```python
from build123d import *

# Parameters (mm, degrees)
BOSS_EXTRUDE1_DEPTH = 30
SKETCH2_R           = 1.5
CUT_EXTRUDE1_DEPTH  = 3
SKETCH3_R           = 1.5
SKETCH3_W           = 15
SKETCH3_H           = 45
CUT_EXTRUDE2_DEPTH  = 3
SKETCH4_W           = 30
SKETCH4_H           = 3
BOSS_EXTRUDE2_DEPTH = 4.75
SKETCH5_R           = 1.5
CUT_EXTRUDE3_DEPTH  = 3
BOSS_EXTRUDE3_DEPTH = 3
BOSS_EXTRUDE4_DEPTH = 3
FILLET1_R           = 1


with BuildPart() as part:
    # Sketch1 → Boss-Extrude1 (new body)
    with BuildSketch(Plane(origin=(0, 0, 0), x_dir=(0, 0, -1), z_dir=(1, 0, 0))):
        Polygon((16.175298805, 7.541832669), (16.175298805, 4.541832669), (-15.824701195, 4.541832669), (-15.824701195, -45.458167331), (-18.824701195, -45.458167331), (-18.824701195, 7.541832669), align=None)
    extrude(amount=-BOSS_EXTRUDE1_DEPTH)

    # Sketch2 → Cut-Extrude1 (cut)
    with BuildSketch(Plane(origin=(0, 7.541832669, 0), x_dir=(1, 0, 0), z_dir=(0, 1, 0))):
        with Locations(Location((-5.5, 12.925298805, 0), (0, 0, 270))):
            Circle(SKETCH2_R)
        with Locations(Location((-24.5, 12.925298805, 0), (0, 0, 270))):
            Circle(SKETCH2_R)
    extrude(amount=-CUT_EXTRUDE1_DEPTH, mode=Mode.SUBTRACT)

    # Sketch3 → Cut-Extrude2 (cut)
    with BuildSketch(Plane.XY.offset(18.824701195)):
        with Locations((-24.5, 2.541832669)):
            Circle(SKETCH3_R)
        with Locations((-5.5, 2.541832669)):
            Circle(SKETCH3_R)
        with Locations((-24.5, -2.458167331)):
            Circle(SKETCH3_R)
        with Locations((-5.5, -2.458167331)):
            Circle(SKETCH3_R)
        with Locations((-24.5, -7.458167331)):
            Circle(SKETCH3_R)
        with Locations((-5.5, -7.458167331)):
            Circle(SKETCH3_R)
        with Locations((-24.5, -12.458167331)):
            Circle(SKETCH3_R)
        with Locations((-5.5, -12.458167331)):
            Circle(SKETCH3_R)
        with Locations((-24.5, -17.458167331)):
            Circle(SKETCH3_R)
        with Locations((-5.5, -17.458167331)):
            Circle(SKETCH3_R)
        with Locations((-24.5, -22.458167331)):
            Circle(SKETCH3_R)
        with Locations((-5.5, -22.458167331)):
            Circle(SKETCH3_R)
        with Locations((-24.5, -27.458167331)):
            Circle(SKETCH3_R)
        with Locations((-5.5, -27.458167331)):
            Circle(SKETCH3_R)
        with Locations((-24.5, -32.458167331)):
            Circle(SKETCH3_R)
        with Locations((-5.5, -32.458167331)):
            Circle(SKETCH3_R)
        with Locations((-24.5, -37.458167331)):
            Circle(SKETCH3_R)
        with Locations((-5.5, -37.458167331)):
            Circle(SKETCH3_R)
        with Locations((-24.5, -42.458167331)):
            Circle(SKETCH3_R)
        with Locations((-5.5, -42.458167331)):
            Circle(SKETCH3_R)
        with Locations((-15, -19.958167331)):
            Rectangle(SKETCH3_W, SKETCH3_H)
    extrude(amount=-CUT_EXTRUDE2_DEPTH, mode=Mode.SUBTRACT)

    # Sketch4 → Boss-Extrude2 (add)
    with BuildSketch(Plane(origin=(0, 0, -16.175298805), x_dir=(-1, 0, 0), z_dir=(0, 0, -1))):
        with Locations((15, 6.041832669)):
            Rectangle(SKETCH4_W, SKETCH4_H)
    extrude(amount=BOSS_EXTRUDE2_DEPTH)

    # Sketch5 → Cut-Extrude3 (cut)
    with BuildSketch(Plane(origin=(0, 7.541832669, 0), x_dir=(1, 0, 0), z_dir=(0, 1, 0))):
        with BuildLine():
            ThreePointArc((-30, 6.925298805), (-25.899494937, 16.824793741), (-16, 20.925298805))
            Line((-16, 20.925298805), (-30, 20.925298805))
            Line((-30, 20.925298805), (-30, 6.925298805))
        make_face()
        with Locations(Location((-15, 17.925298805, 0), (0, 0, 270))):
            Circle(SKETCH5_R)
        with BuildLine():
            Line((0, 20.925298805), (-14, 20.925298805))
            ThreePointArc((-14, 20.925298805), (-4.100505063, 16.824793741), (0, 6.925298805))
            Line((0, 6.925298805), (0, 20.925298805))
        make_face()
    extrude(amount=-CUT_EXTRUDE3_DEPTH, mode=Mode.SUBTRACT)

    # Sketch6 → Boss-Extrude3 (add)
    with BuildSketch(Plane(origin=(0, 0, 0), x_dir=(0, 0, -1), z_dir=(1, 0, 0))):
        Polygon((-15.824701195, 4.541832669), (-5.824701195, 4.541832669), (-15.824701195, -5.458167331), align=None)
    extrude(amount=-BOSS_EXTRUDE3_DEPTH)

    # Sketch7 → Boss-Extrude4 (add)
    with BuildSketch(Plane.ZY.offset(30)):
        Polygon((5.824701195, 4.541832669), (15.824701195, -5.458167331), (15.824701195, 4.541832669), align=None)
    extrude(amount=-BOSS_EXTRUDE4_DEPTH)

    # Fillet1
    fillet1_edges = [part.edges().sort_by_distance(p)[0] for p in [
        (-3, -0.458167331, 15.824701195),
        (-1.5, -5.458167331, 15.824701195),
        (-3, 4.541832669, 10.824701195),
        (-1.5, 4.541832669, 5.824701195),
        (-27, 4.541832669, 10.824701195),
        (-28.5, 4.541832669, 5.824701195),
        (-27, -0.458167331, 15.824701195),
        (-28.5, -5.458167331, 15.824701195),
    ]]
    fillet(fillet1_edges, radius=FILLET1_R - 0.0001)  # a hair under: the kernel refuses the full size


solid = part.part
```
For this review, take the finished solid that the model builds, in its own axes (mm). A direction names the side the tool comes from. Coordinates: 2 decimals unless noted, no trailing zeros. Order: outer loops, then holes, each group sorted by start corner. A loop starts at its lowest first (then second) coordinate and runs counter-clockwise, first axis right, second up. Notation, with made-up numbers: (-10.5, 14.5) -> (21.5, 14.5) arc R34 cw to (21.5, 51.5) -> close; hole circle Ø1 at (-16, 30). An arc over 180 degrees is marked (long way). Use CSV: the item, a comma, the result in double quotes. Start each with the question number.
Item 1: For faces 4 (the face through (-26.008, 6.063, -16.715)), 5 (the face through (-15, -42.458, 17)), 6 (the face through (-15, 4.542, -2)), list the 3-axis set-ups (+Z, -Z, +X, -X, +Y, -Y) from which the entire face can be reached by the end or side of a thin tool; tool diameter is ignored.
Item 2: We need section B-B, the plane x = -20. Give the boundary of the cut face in (y, z), then the cut area to 3 significant figures.
Item 3: We need section A-A, the plane x = -15. Give the boundary of the cut face in (y, z).
Item 4: Insertion check: pin 1 (15 mm diameter, centred on x = -21, y = -26.5, fed in from -Z); pin 2 (8 mm diameter, centred on x = -26, z = -8.5, fed in from -Y). Each pin has a flat end and moves straight along its axis. Give the tip position at first contact, or say it passes through.
Item 5: Draft analysis for pull direction X (two halves, no side actions). For faces 1 (the face through (-25.69, -43.37, 17.35)), 2 (the face through (-15, -45.458, 17)), 3 (the face through (-30, -9, 16)), state which applies: pulls with the +X half, pulls with the -X half, needs draft (parallel to the pull), parting line crosses it, or undercut.
Item 6: We need section D-D, the plane x = -24.5. Give the number of separate pieces and of enclosed holes in the cut face, then the cut area to 3 significant figures.
Item 7: Wall thickness on probe 1 along X at (y, z) = (1, 9.5); probe 2 along Z at (x, y) = (-1.5, -23.5); probe 3 along Y at (x, z) = (-28, -6): over which ranges is each line inside the solid? List them lowest first.
Item 8: We need section C-C, the plane z = 10. Give the boundary of the cut face in (x, y).
Derived:
1,face 4,"-Z, -X, +Y, -Y"
1,face 5,"+Z, -Z"
1,face 6,"-Z, -Y"
2,outline,"(-45.46, 15.82) -> (-42.46, 15.82) -> (-42.46, 18.82) -> (-45.46, 18.82) -> close; (2.54, 15.82) -> (4.54, 15.82) -> (4.54, -20.34) -> (7.54, -20.34) -> (7.54, 18.82) -> (2.54, 18.82) -> close"
2,area,"132 mm^2"
3,outline,"(-45.46, 15.82) -> (-42.46, 15.82) -> (-42.46, 18.82) -> (-45.46, 18.82) -> close; (2.54, 15.82) -> (4.54, 15.82) -> (4.54, -16.43) -> (7.54, -16.43) -> (7.54, 18.82) -> (2.54, 18.82) -> close; (4.54, -20.93) -> (7.54, -20.93) -> (7.54, -19.43) -> (4.54, -19.43) -> close"
4,pin 1,"stops at z = 15.82"
4,pin 2,"stops at y = 4.54"
5,face 1,"undercut"
5,face 2,"needs draft"
5,face 3,"pulls with the -X half"
6,separate pieces,"12"
6,enclosed holes,"0"
6,area,"162 mm^2"
7,probe 1,"x = -30 to -27, -3 to 0"
7,probe 2,"z = 15.82 to 18.82"
7,probe 3,"y = 4.54 to 7.54"
8,outline,"(-30, 0.37) -> (-27, 0.37) -> (-27, 3.54) arc R1 cw to (-26, 4.54) -> (-4, 4.54) arc R1 cw to (-3, 3.54) -> (-3, 0.37) -> (0, 0.37) -> (0, 7.54) -> (-30, 7.54) -> close"
